For this review, take the finished solid that the model builds, in its own axes (mm). Coordinates: 2 decimals unless noted, no trailing zeros. Use one line per item in the form item = value. Start each with the question number.
1. For pin 1 Ø4 at (x, y) = (121, 275.5) entering from -Z, flat-tipped, find the tip position at first contact; note if it passes through.
2. Draft analysis for pull direction X (two halves, no side actions). For faces 1 (the face through (-37.43, -15.04, 2.54)), 2 (the face through (280.86, -15.35, 2.54)), 3 (the face through (120, 146, 0)), state which applies: +X half, -X half, draft (parallel to the pull), parting line (faces both ways), or undercut.
3. To check wall thickness, follow probe 1 along X at (y, z) = (-6, 2.95). State the ranges of the line that lie inside material, in increasing order.
```python
from build123d import *

# Parameters (mm, degrees)
SKETCH_1_W          = 330
SKETCH_1_H          = 330
EXTRUDE_1_DEPTH     = 5
FILLET_1_R          = 20
SKETCH_2_R          = 3.3
CUT_EXTRUDE_1_DEPTH = 10


with BuildPart() as part:
    # 草图1 → 凸台-拉伸1 (new body)
    with BuildSketch(Plane.XY):
        with Locations((121.871247651, 143.942488789)):
            Rectangle(SKETCH_1_W, SKETCH_1_H)
    extrude(amount=EXTRUDE_1_DEPTH)

    # 圆角1
    fillet_1_edges = [part.edges().sort_by_distance(p)[0] for p in [
        (-43.128752349, 308.942488789, 2.5),
        (286.871247651, 308.942488789, 2.5),
        (286.871247651, -21.057511211, 2.5),
        (-43.128752349, -21.057511211, 2.5),
    ]]
    fillet(fillet_1_edges, radius=FILLET_1_R)

    # 草图2 → 切除-拉伸1 (cut)
    with BuildSketch(Plane(origin=(0, 0, 0), x_dir=(-1, 0, 0), z_dir=(0, 0, -1))):
        with Locations((28.128752349, -6.057511211)):
            Circle(SKETCH_2_R)
        with Locations((-271.871247651, -6.057511211)):
            Circle(SKETCH_2_R)
        with Locations((-271.871247651, 293.942488789)):
            Circle(SKETCH_2_R)
        with Locations((28.128752349, 293.942488789)):
            Circle(SKETCH_2_R)
    extrude(amount=-CUT_EXTRUDE_1_DEPTH, mode=Mode.SUBTRACT)


solid = part.part
```
Conclusion:
q1.pin_1 = 0
q2.face_1 = -X half
q2.face_2 = +X half
q2.face_3 = draft
q3.probe_1 = -42.51 to -31.43, -24.83 to 268.57, 275.17 to 286.25
